The listing builds one solid part. Answer for the finished solid, in the listing's coordinates (mm). A direction names the side the tool comes from. Coordinates: 2 decimals unless noted, no trailing zeros. Order: outer loops, then holes, each group sorted by start corner. A loop starts at its lowest first (then second) coordinate and runs counter-clockwise, first axis right, second up. Notation, with made-up numbers: (55, 51.25) -> (81, 51.25) arc R26 ccw to (81, 73.25) -> close; hole circle Ø1 at (87, 3). An arc over 180 degrees is marked (long way). Answer in a Markdown table with one row per item. Add a question column.
```python
from build123d import *

# Parameters (mm, degrees)
SKETCH1_R           = 1
SKETCH1_R_2         = 4.25
BOSS_EXTRUDE1_DEPTH = 10
FILLET1_R           = 5


with BuildPart() as part:
    # Sketch1 → Boss-Extrude1 (new body)
    with BuildSketch(Plane.XY):
        with BuildLine():
            Line((-22.1, 10), (-10.782884141, 10))
            Line((-10.782884141, 10), (-10.782884141, 47.312260738))
            ThreePointArc((-10.782884141, 47.312260738), (0, 58.095144879), (10.782884141, 47.312260738))
            Line((10.782884141, 47.312260738), (10.782884141, 10))
            Line((10.782884141, 10), (22.1, 10))
            ThreePointArc((22.1, 10), (32.1, 0), (22.1, -10))
            Line((22.1, -10), (10, -10))
            Line((10, -10), (10, -80))
            Line((10, -80), (10.352856736, -132.530872001))
            ThreePointArc((10.352856736, -132.530872001), (0, -143.041784363), (-10.352856736, -132.530872001))
            Line((-10.352856736, -132.530872001), (-10, -80))
            Line((-10, -80), (-10, -10))
            Line((-10, -10), (-22.1, -10))
            ThreePointArc((-22.1, -10), (-32.1, 0), (-22.1, 10))
        make_face()
        with Locations((-22.1, 0)):
            Circle(SKETCH1_R, mode=Mode.SUBTRACT)
        with Locations((22.1, 0)):
            Circle(SKETCH1_R, mode=Mode.SUBTRACT)
        with Locations((0, -80)):
            Circle(SKETCH1_R, mode=Mode.SUBTRACT)
        with Locations((0, 47.312260738)):
            Circle(SKETCH1_R_2, mode=Mode.SUBTRACT)
        with Locations((0, -132.687739262)):
            Circle(SKETCH1_R_2, mode=Mode.SUBTRACT)
    extrude(amount=BOSS_EXTRUDE1_DEPTH)

    # Fillet1
    fillet1_edges = [part.edges().sort_by_distance(p)[0] for p in [
        (-10.782884141, 10, 5),
        (10.782884141, 10, 5),
        (10, -10, 5),
        (-10, -10, 5),
    ]]
    fillet(fillet1_edges, radius=FILLET1_R)


solid = part.part
```
Q1. For faces 5 (the face through (10.783, 31, 5)), 6 (the face through (19, -10, 5)), 7 (the face through (10, -47, 5)), 8 (the face through (-12, -11, 5)), 9 (the face through (-19, 10, 5)), determine the directions among +Z, -Z, +X, -X, +Y, -Y from which every point of the face is accessible in a straight line to the end or side of a thin tool.
Q2. A cutting plane is placed at B-B (y = -22). Determine the outline of the cut face in (x, z).
Q3. A cutting plane is placed at C-C (x = -6). Determine the outline of the cut face in (y, z).
Q4. A cutting plane is placed at A-A (z = 3.25). Determine the outline of the cut face in (x, y).
Q5. Given pin 1 (3 mm diameter, centred on y = 25.5, z = 4, fed in from -X); pin 2 (2 mm diameter, centred on x = -5, z = 3, fed in from -Y); pin 3 (3 mm diameter, centred on x = -19.5, z = 6.5, fed in from +Y), each flat-ended and moving along its own axis, determine where each tip first touches the part or whether it passes through.
Q6. Determine the mould class of faces 1 (the face through (-10.783, 31, 5)), 2 (the face through (-0.921, -136.837, 4.93)), 3 (the face through (12, -11, 5)), 4 (the face through (-0.921, 43.163, 4.93)) for opening direction X: +X half, -X half, draft (parallel to the pull), parting line (faces both ways), or undercut.
Q7. Straight lines are drawn through the part: line 1 (Y direction, x = 0, z = 5); line 2 (Y direction, x = -2.5, z = 5.75); line 3 (X direction, y = 19, z = 2.5). For each, find the intervals that lie inside material, in ascending order.
Returned:
| question | item | result |
|---|---|---|
| 1 | face 5 | +Z, -Z, +X, +Y |
| 1 | face 6 | +Z, -Z, +X, -Y |
| 1 | face 7 | +Z, -Z, +X |
| 1 | face 8 | +Z, -Z, -X |
| 1 | face 9 | +Z, -Z, -X, +Y |
| 2 | outline | (-10, 0) -> (10, 0) -> (10, 10) -> (-10, 10) -> close |
| 3 | outline | (-141.13, 0) -> (56.27, 0) -> (56.27, 10) -> (-141.13, 10) -> close |
| 4 | outline | (-22.1, -10) -> (-15, -10) arc R5 cw to (-10, -15) -> (-10, -80) -> (-10.35, -132.53) arc R10.35 ccw (long way) to (10.35, -132.53) -> (10, -80) -> (10, -15) arc R5 cw to (15, -10) -> (22.1, -10) arc R10 ccw to (22.1, 10) -> (15.78, 10) arc R5 cw to (10.78, 15) -> (10.78, 47.31) arc R10.78 ccw to (-10.78, 47.31) -> (-10.78, 15) arc R5 cw to (-15.78, 10) -> (-22.1, 10) arc R10 ccw to start; hole circle Ø2 at (-22.1, 0); hole circle Ø8.5 at (0, -132.69); hole circle Ø8.5 at (0, 47.31); hole circle Ø2 at (0, -80); hole circle Ø2 at (22.1, 0) |
| 5 | pin 1 | stops at x = -10.78 |
| 5 | pin 2 | stops at y = -142.24 |
| 5 | pin 3 | stops at y = 10 |
| 6 | face 1 | -X half |
| 6 | face 2 | undercut |
| 6 | face 3 | +X half |
| 6 | face 4 | undercut |
| 7 | line 1 | y = -143.04 to -136.94, -128.44 to -81, -79 to 43.06, 51.56 to 58.1 |
| 7 | line 2 | y = -142.74 to -136.12, -129.25 to 43.88, 50.75 to 57.8 |
| 7 | line 3 | x = -10.78 to 10.78 |
